Verification items for this drawing (mm, ordinates from the low corner). A direction names the side the tool comes from. Give positions to 0.01 mm unless a question says otherwise; leave off trailing zeros. Loops run counter-clockwise (first coordinate to the right, second up) from the corner with the lowest first, then second, coordinate; pieces in that order, holes last. Notation, with made-up numbers: (80.5, 16) -> (131.5, 16) arc R29 cw to (131.5, 46) -> close; hole circle Ø7 at (-1.75, -19.75). An arc over 180 degrees is marked (long way). Write item = value, one per line.
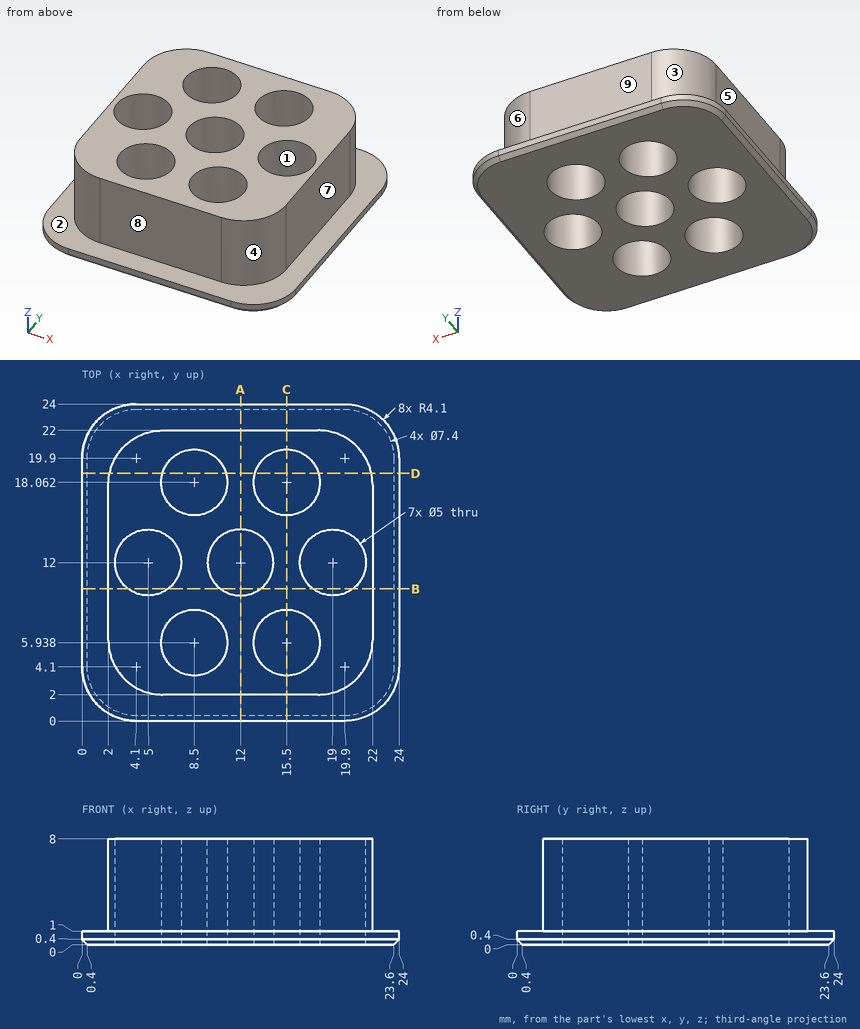
Item 1: Thickness scan on L1, parallel to Y at x = 15.5, z = 3.75; L2, parallel to X at y = 12.75, z = 5 (1 decimal); L3, parallel to X at y = 13.75, z = 7.75 (1 decimal). Record the ranges inside material, lowest first. Write a range as [from, to].
Answer:
L1 = [2, 3.44], [8.44, 15.56], [20.56, 22]
L2 = [2, 2.6], [7.4, 9.6], [14.4, 16.6], [21.4, 22]
L3 = [2, 3.2], [6.8, 10.2], [13.8, 17.2], [20.8, 22]
Item 2: Section check A-A, the plane x = 12. Record the cut outline in (y, z), plus the area to 3 significant figures.
Answer:
outline = (0, 0.4) -> (0.4, 0) -> (9.5, 0) -> (9.5, 8) -> (2, 8) -> (2, 1) -> (0, 1) -> close; (14.5, 0) -> (23.6, 0) -> (24, 0.4) -> (24, 1) -> (22, 1) -> (22, 8) -> (14.5, 8) -> close
area = 124 mm^2
Item 3: Gauge pin test, flat ends, axial feed: pin 1 (12 mm diameter, centred on x = 10.5, y = 13, fed in from +Z); pin 2 (3.5 mm diameter, centred on x = 11, z = 6, fed in from -Y); pin 3 (3 mm diameter, centred on y = 21.5, z = 6.5, fed in from +X). Record the tip position at first contact, or that the pin passes through.
Answer:
pin_1 = 8
pin_2 = 2
pin_3 = 21.42
Item 4: Section check B-B, the plane y = 10. Record the cut outline in (x, z).
Answer:
outline = (0, 0.4) -> (0.4, 0) -> (3.5, 0) -> (3.5, 8) -> (2, 8) -> (2, 1) -> (0, 1) -> close; (6.5, 0) -> (10.5, 0) -> (10.5, 8) -> (6.5, 8) -> close; (13.5, 0) -> (17.5, 0) -> (17.5, 8) -> (13.5, 8) -> close; (20.5, 0) -> (23.6, 0) -> (24, 0.4) -> (24, 1) -> (22, 1) -> (22, 8) -> (20.5, 8) -> close
Item 5: Tool access check on the marked faces 5, 6, 7, 8 and 9. Record the directions out of +Z, -Z, +X, -X, +Y, -Y that give a thin tool (end or side, any length) a straight path to the whole face; none if there is none.
Answer:
face_5 = +Z, -X, +Y, -Y
face_6 = +Z, +X, +Y
face_7 = +Z, +X, +Y, -Y
face_8 = +Z, +X, -X, -Y
face_9 = +Z, +X, -X, +Y
Item 6: Section check C-C, the plane x = 15.5. Record the cut outline in (y, z).
Answer:
outline = (0, 0.4) -> (0.4, 0) -> (3.44, 0) -> (3.44, 8) -> (2, 8) -> (2, 1) -> (0, 1) -> close; (8.44, 0) -> (15.56, 0) -> (15.56, 8) -> (8.44, 8) -> close; (20.56, 0) -> (23.6, 0) -> (24, 0.4) -> (24, 1) -> (22, 1) -> (22, 8) -> (20.56, 8) -> close
Item 7: Draft check along Y on the marked faces 1, 2, 3 and 4. Enter one of: +Y half, -Y half, draft (parallel to the pull), parting line (faces both ways), or undercut.
Answer:
face_1 = undercut
face_2 = draft
face_3 = +Y half
face_4 = -Y half
Item 8: Section check D-D, the plane y = 18.75. Record the cut outline in (x, z), plus the area to 3 significant figures.
Answer:
outline = (0, 0.4) -> (0.4, 0) -> (6.1, 0) -> (6.1, 8) -> (2.09, 8) -> (2.09, 1) -> (0, 1) -> close; (10.9, 0) -> (13.1, 0) -> (13.1, 8) -> (10.9, 8) -> close; (17.9, 0) -> (23.6, 0) -> (24, 0.4) -> (24, 1) -> (21.91, 1) -> (21.91, 8) -> (17.9, 8) -> close
area = 85.7 mm^2
